Here's how the part is built. I have some questions about the finished solid (model axes, mm). A direction names the side the tool comes from. Coordinates: 2 decimals unless noted, no trailing zeros. Loops run counter-clockwise (first coordinate to the right, second up) from the corner with the lowest first, then second, coordinate; pieces in that order, holes last. Notation, with made-up numbers: M -11,49.5 L 43,49.5 A12 ccw 43,66.5 Z; hole C -35.5,56.25 d8. An arc over 180 degrees is marked long. Use one line per item in the form item = value. Start each with the question number.
(1) On a 3-axis mill with a long thin cutter (end or side, diameter ignored), from which of +Z, -Z, +X, -X, +Y, -Y can I reach the whole of each face in a straight line? I mean faces 4 (the cylindrical face through (4.93, -1.07, -69.75)), 5 (the flat face through (22, 4, -81)), 6 (the flat face through (21.911, 6, -29)). Say none if no direction works.
(2) Please list where these lines run through material, in increasing order: L1, parallel to X at y = 9, z = -78; L2, parallel to Y at x = 24, z = -86; L3, parallel to X at y = 11, z = -36.
(3) Imagine slicing it at B-B, the plane z = -23. Please give me the cut outline in (x, y).
(4) Will these pins go through, and if not, where does the flat tip stop? P1, Ø9.5, axis at x = 23.5, z = -38, coming from the -Y side; P2, Ø6, axis at x = 10, y = 2, coming from the -Z side; P3, Ø1, axis at x = 28, y = -10.5, coming from the -Z side.
(5) Thinking about a two-plate mould opening in Y: for faces 1 (the cylindrical face through (16.13, 6.08, -10.09)), 2 (the flat face through (23, 0, -33)), 3 (the cylindrical face through (26.93, -3.78, -80.05)), which applies, +Y half, -Y half, draft (parallel to the pull), parting line (faces both ways), or undercut?
(6) Imagine slicing it at A-A, the plane y = 6. Please give me the cut outline in (x, z), and give its area (3 significant figures).
(7) Imagine slicing it at D-D, the plane x = 15. Please give me the cut outline in (y, z).
(8) Imagine slicing it at C-C, the plane z = -82. Please give me the cut outline in (x, y), and give its area (3 significant figures).
```python
from build123d import *

# Parameters (mm, degrees)
F0_R     = 6
F1_DEPTH = 32
F2_W     = 12
F2_H     = 6.026334
F2_W_2   = 11.82259
F2_H_2   = 25
F2_H_3   = 33.973666
F3_DEPTH = 20


with BuildPart() as f1:
    # F0 (on Right) → F1 (new body)
    with BuildSketch(Plane.YZ):
        with BuildLine():
            Line((12, 0), (0, 0))
            Line((0, 0), (0, -67.026334))
            ThreePointArc((0, -67.026334), (-1.098095, -69.779323), (-3.789474, -71.02079))
            ThreePointArc((-3.789474, -71.02079), (-13.323708, -96.882144), (12, -86))
            Line((12, -86), (12, 0))
        make_face()
        with Locations((-3, -86)):
            Circle(F0_R, mode=Mode.SUBTRACT)
    extrude(amount=F1_DEPTH)

    # F2 (on face) → F3 (cut, symmetric)
    with BuildSketch(Plane.XZ):
        with Locations((16, -64.013167)):
            Rectangle(F2_W, F2_H)
        with BuildLine():
            ThreePointArc((10.088705, -41), (16, -46.911295), (21.911295, -41))
            Line((21.911295, -41), (10.088705, -41))
        make_face()
        with Locations((16, -28.5)):
            Rectangle(F2_W_2, F2_H_2)
        with BuildLine():
            Line((10.088705, -16), (21.911295, -16))
            ThreePointArc((21.911295, -16), (16, -10.088705), (10.088705, -16))
        make_face()
        with BuildLine():
            ThreePointArc((16, 0), (27.313708, -4.686292), (32, -16))
            Line((32, -16), (32, 0))
            Line((32, 0), (16, 0))
        make_face()
        with BuildLine():
            Line((0, 0), (0, -16))
            ThreePointArc((0, -16), (4.686292, -4.686292), (16, 0))
            Line((16, 0), (0, 0))
        make_face()
        with Locations((16, -84.013167)):
            Rectangle(F2_W, F2_H_3)
    extrude(amount=F3_DEPTH, both=True, mode=Mode.SUBTRACT)


solid = f1.part
```
Answer:
q1.face_4 = +Z, +X, -X, -Y
q1.face_5 = -Z, +Y, -Y
q1.face_6 = +Y, -Y
q2.L1 = 0 to 10, 22 to 32
q2.L2 = -18 to -9, 3 to 12
q2.L3 = 0 to 10.09, 21.91 to 32
q3.outline = M 0,0 L 10.09,0 L 10.09,12 L 0,12 Z; M 21.91,0 L 32,0 L 32,12 L 21.91,12 Z
q4.P1 = 0
q4.P2 = -100.87
q4.P3 = -99.27
q5.face_1 = draft
q5.face_2 = -Y half
q5.face_3 = undercut
q6.outline = M 0,-98 L 10,-98 L 10,-61 L 22,-61 L 22,-98 L 32,-98 L 32,-16 A16 ccw 16,0 A16 ccw 0,-16 Z; hole M 10.09,-41 A5.91 ccw 21.91,-41 L 21.91,-16 A5.91 ccw 10.09,-16 Z
q6.area = 2,180 mm²
q7.outline = M 0,-61 L 12,-61 L 12,-46.83 L 0,-46.83 Z; M 0,-10.17 L 12,-10.17 L 12,-0.03 L 0,-0.03 Z
q8.outline = M 0,-17.46 L 10,-17.46 L 10,-7.47 L 0,-7.47 Z; M 0,1.47 L 10,1.47 L 10,12 L 0,12 Z; M 22,-17.46 L 32,-17.46 L 32,-7.47 L 22,-7.47 Z; M 22,1.47 L 32,1.47 L 32,12 L 22,12 Z
q8.area = 410 mm²
